```python
from build123d import *

# Parameters (mm, degrees)
SKETCH1_W           = 254
SKETCH1_H           = 33
BOSS_EXTRUDE1_DEPTH = 0.2
BOSS_EXTRUDE2_DEPTH = 254


with BuildPart() as part:
    # Sketch1 → Boss-Extrude1 (new body)
    with BuildSketch(Plane(origin=(0, 0, 0), x_dir=(1, 0, 0), z_dir=(0, 1, 0))):
        with Locations((-6.018162295, 0)):
            Rectangle(SKETCH1_W, SKETCH1_H)
    extrude(amount=BOSS_EXTRUDE1_DEPTH)

    # Sketch4 → Boss-Extrude2 (add)
    with BuildSketch(Plane(origin=(-133.018162295, 0, 0), x_dir=(0, 0, -1), z_dir=(1, 0, 0))):
        with BuildLine():
            Line((16.5, 0.2), (16.5, 3.005611905))
            ThreePointArc((16.5, 3.005611905), (17.439298034, 3.944909939), (16.5, 4.884207973))
            Line((16.5, 4.884207973), (16.5, 9.2))
            Line((16.5, 9.2), (16.406492637, 9.371049015))
            add(Edge.make_bspline(
                [(16.406492637, 9.371049015), (15.606591952, 9.884020198), (14.657842295, 10.216248434), (13.711270965, 10.299814324)],
                knots=[0, 0, 0, 0, 1, 1, 1, 1], degree=3))
            Line((13.711270965, 10.299814324), (13.693401418, 10.097401579))
            add(Edge.make_bspline(
                [(16.2968, 9.2), (15.089651085, 9.974136863), (13.693401418, 10.097401579)],
                knots=[0, 0, 0, 1, 1, 1], degree=2))
            Line((16.2968, 9.2), (16.2968, 4.652405576))
            ThreePointArc((16.2968, 4.652405576), (17.236098034, 3.944909939), (16.2968, 3.237414303))
            Line((16.2968, 3.237414303), (16.2968, 0.2))
            Line((16.2968, 0.2), (16.5, 0.2))
        make_face()
    boss_extrude2 = extrude(amount=BOSS_EXTRUDE2_DEPTH)

    # Mirror1: Boss-Extrude2 across plane
    add(boss_extrude2.mirror(Plane.XY))


solid = part.part
```
Input: part model. Units: mm. Frame: model coordinates. Coordinates: 2 decimals unless noted, no trailing zeros.
1) Pin query (flat end, axial travel): pin 1 Ø2 at (x, y) = (-5.5, 2.5) entering from +Z; pin 2 Ø4.5 at (x, y) = (-66, 7.5) entering from -Z; pin 3 Ø4 at (x, y) = (47, 5) entering from +Z; pin 4 Ø3.5 at (x, y) = (43, 1) entering from +Z. Return the tip coordinate at first contact, or that it passes through.
2) Material intervals for line 1 along Z through (x, y) = (-8, 5.75); line 2 along Z through (x, y) = (73, 3.75); line 3 along Y through (x, z) = (-42, 1.5), sorted ascending.
3) Mould query, pull axis Z, two halves, no side actions, for faces 1 (the flat face through (-8, 7, -16.5)), 2 (the flat face through (-8, 7, 16.297)), 3 (the flat face through (-8, 7, 16.5)), 4 (the flat face through (-8, 0, 0)). Classes: pulls with the +Z half, pulls with the -Z half, needs draft (parallel to the pull), parting line crosses it, or undercut.
Check result:
1. pin 1: stops at z = 17.33
1. pin 2: stops at z = -16.5
1. pin 3: stops at z = 17.44
1. pin 4: stops at z = 16.5
2. line 1: z = -16.5 to -16.3, 16.3 to 16.5
2. line 2: z = -17.42 to -17.21, 17.21 to 17.42
2. line 3: y = 0 to 0.2
3. face 1: pulls with the -Z half
3. face 2: undercut
3. face 3: pulls with the +Z half
3. face 4: needs draft
